from build123d import *

# Parameters (mm, degrees)
F0_W     = 64
F0_H     = 54
F0_W_2   = 60
F0_H_2   = 50
F0_R     = 3.25
F1_DEPTH = 2
F2_W     = 64
F2_H     = 54
F2_W_2   = 60
F2_H_2   = 50
F3_DEPTH = 20


with BuildPart() as f1:
    # F0 (on Top) → F1 (new body)
    with BuildSketch(Plane.XY):
        Rectangle(F0_W, F0_H)
        Rectangle(F0_W_2, F0_H_2, mode=Mode.SUBTRACT)
        Rectangle(F0_W_2, F0_H_2)
        with Locations((-20, -15)):
            Circle(F0_R, mode=Mode.SUBTRACT)
        with Locations((0, -15)):
            Circle(F0_R, mode=Mode.SUBTRACT)
        with Locations((20, -15)):
            Circle(F0_R, mode=Mode.SUBTRACT)
        with Locations((-20, 15)):
            Circle(F0_R, mode=Mode.SUBTRACT)
        with Locations((0, 15)):
            Circle(F0_R, mode=Mode.SUBTRACT)
        with Locations((20, 15)):
            Circle(F0_R, mode=Mode.SUBTRACT)
    extrude(amount=F1_DEPTH)

    # F2 (on face) → F3 (join)
    with BuildSketch(Plane.XY.offset(2)):
        Rectangle(F2_W, F2_H)
        Rectangle(F2_W_2, F2_H_2, mode=Mode.SUBTRACT)
    extrude(amount=F3_DEPTH)


solid = f1.part
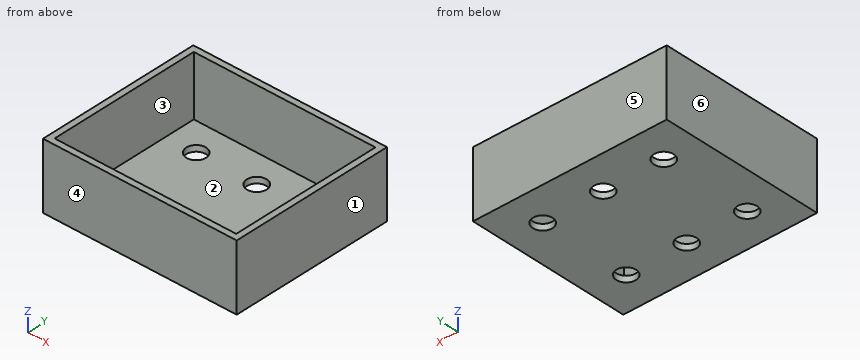
CAD build for the part. Positions are in the model's coordinates, mm. Face numbers are marked on the shaded views. A direction names the side the tool comes from. Give positions to 0.01 mm unless a question says otherwise; leave off trailing zeros. Order: outer loops, then holes, each group sorted by start corner. A loop starts at its lowest first (then second) coordinate and runs counter-clockwise, first axis right, second up. Notation, with made-up numbers: (61.25, 86.5) -> (73.25, 86.5) arc R19 ccw to (73.25, 91.5) -> close; hole circle Ø5 at (41.25, 75.5). An arc over 180 degrees is marked (long way). Return JSON: item names as keys, results as strings.
Q1. Mould opens along Y. For the marked faces 3, 4, 5 and 6 say: pulls with the +Y half, pulls with the -Y half, needs draft (parallel to the pull), parting line crosses it, or undercut.
Working result:
{"face 3": "undercut", "face 4": "pulls with the -Y half", "face 5": "pulls with the +Y half", "face 6": "needs draft"}
Q2. Saw through at B-B (z = 16.5). Write the cut outline in (x, y), then the cut area to 3 significant figures.
Working result:
{"outline": "(-32, -27) -> (32, -27) -> (32, 27) -> (-32, 27) -> close; hole (-30, -25) -> (30, -25) -> (30, 25) -> (-30, 25) -> close", "area": "456 mm²"}
Q3. Saw through at D-D (x = -11). Write the cut outline in (y, z), then the cut area to 3 significant figures.
Working result:
{"outline": "(-27, 0) -> (27, 0) -> (27, 22) -> (25, 22) -> (25, 2) -> (-25, 2) -> (-25, 22) -> (-27, 22) -> close", "area": "188 mm²"}
Q4. Which spindle directions (+Z, -Z, +X, -X, +Y, -Y) get a long thin tool onto all of the face, cutting with end or side? Do the marked faces 1 and 2. Say none if no direction does.
Working result:
{"face 1": "+Z, -Z, +X, +Y, -Y", "face 2": "+Z"}
Q5. Flat gauge pins, fed straight in: pin 1 (7.5 mm diameter, centred on x = 0, y = 15, fed in from -Z); pin 2 (10.5 mm diameter, centred on x = 20, y = 15, fed in from +Z). Where does each tip first touch, or does it go through?
Working result:
{"pin 1": "z = 0", "pin 2": "z = 2"}
Q6. Saw through at C-C (x = -20). Write the cut outline in (y, z), then the cut area to 3 significant figures.
Working result:
{"outline": "(-27, 0) -> (-18.25, 0) -> (-18.25, 2) -> (-25, 2) -> (-25, 22) -> (-27, 22) -> close; (-11.75, 0) -> (11.75, 0) -> (11.75, 2) -> (-11.75, 2) -> close; (18.25, 0) -> (27, 0) -> (27, 22) -> (25, 22) -> (25, 2) -> (18.25, 2) -> close", "area": "162 mm²"}
Q7. Drill centre lines: line 1 (Y direction, x = -20, z = 0.8); line 2 (Y direction, x = -16, z = 20.75); line 3 (X direction, y = 4, z = 21). Where is each one in solid material? Low to high.
Working result:
{"line 1": "-27 to -18.25, -11.75 to 11.75, 18.25 to 27", "line 2": "-27 to -25, 25 to 27", "line 3": "-32 to -30, 30 to 32"}
Q8. Saw through at A-A (y = 15). Write the cut outline in (x, z).
Working result:
{"outline": "(-32, 0) -> (-23.25, 0) -> (-23.25, 2) -> (-30, 2) -> (-30, 22) -> (-32, 22) -> close; (-16.75, 0) -> (-3.25, 0) -> (-3.25, 2) -> (-16.75, 2) -> close; (3.25, 0) -> (16.75, 0) -> (16.75, 2) -> (3.25, 2) -> close; (23.25, 0) -> (32, 0) -> (32, 22) -> (30, 22) -> (30, 2) -> (23.25, 2) -> close"}
